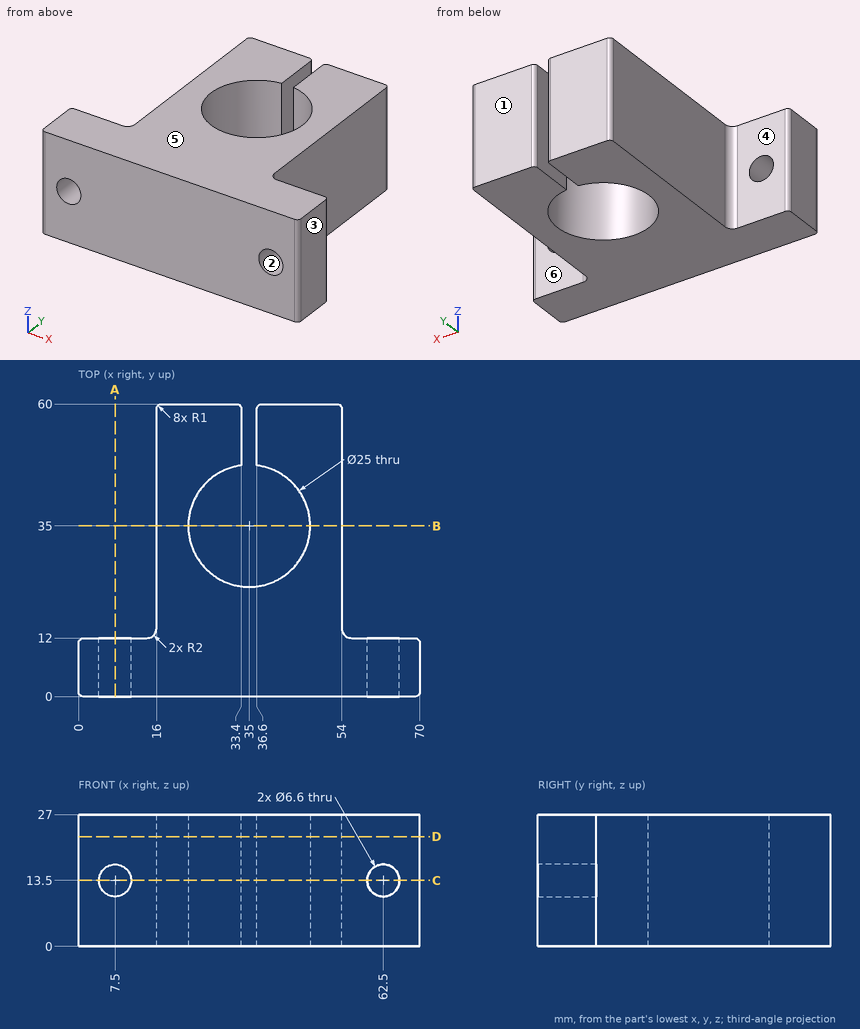
Study the drawing (mm; zero at the part's minimum x, y, z) and answer. A direction names the side the tool comes from. Give positions to 0.01 mm unless a question says otherwise; leave off trailing zeros. Loops run counter-clockwise (first coordinate to the right, second up) from the corner with the lowest first, then second, coordinate; pieces in that order, holes last. Notation, with made-up numbers: (55.25, 68.25) -> (75.25, 68.25) arc R19 ccw to (75.25, 79.25) -> close; hole circle Ø11 at (-36.5, 70). An arc over 180 degrees is marked (long way). Use a Markdown table: item, result. Add a question column.
1) The part is cut by section D-D, the plane z = 22.5. Determine the outline of the cut face in (x, y), plus the area to 3 significant figures.
2) The part is cut by section A-A, the plane x = 7.5. Determine the outline of the cut face in (y, z), plus the area to 3 significant figures.
3) The part is cut by section C-C, the plane z = 13.5. Count the separate pieces of the cut face and the enclosed holes in it, plus the area to 3 significant figures.
4) Each of these flat-tipped pins is pushed along its axis until it touches: P1, Ø5, axis at y = 17, z = 6, coming from the -X side; P2, Ø22.5, axis at x = 35, y = 35, coming from the +Z side; P3, Ø4, axis at x = 8, z = 18.5, coming from the +Y side; P4, Ø9.5, axis at y = 51.5, z = 13.5, coming from the +X side. Where does it stop, or does it pass through?
5) Which of the six approach directions +Z, -Z, +X, -X, +Y, -Y give full straight-line access (tool end or side, diameter ignored) to the marked faces 4, 5 and 6?
6) Consider line 1 along X through (y, z) = (4.25, 13.5); line 2 along X through (y, z) = (51, 6); line 3 along X through (y, z) = (7.5, 11.5). Determine where each line is inside the solid, lowest interval first.
7) The part is cut by section B-B, the plane y = 35. Determine the outline of the cut face in (x, z).
8) For a pull along X with two mould halves and no side action, classify the marked faces 1, 2 and 3 as +X half, -X half, draft (parallel to the pull), parting line (faces both ways), or undercut.
Reported:
| question | item | result |
|---|---|---|
| 1 | outline | (0, 1) arc R1 ccw to (1, 0) -> (69, 0) arc R1 ccw to (70, 1) -> (70, 11) arc R1 ccw to (69, 12) -> (56, 12) arc R2 cw to (54, 14) -> (54, 59) arc R1 ccw to (53, 60) -> (37.6, 60) arc R1 ccw to (36.6, 59) -> (36.6, 47.4) arc R12.5 cw (long way) to (33.4, 47.4) -> (33.4, 59) arc R1 ccw to (32.4, 60) -> (17, 60) arc R1 ccw to (16, 59) -> (16, 14) arc R2 cw to (14, 12) -> (1, 12) arc R1 ccw to (0, 11) -> close |
| 1 | area | 2,130 mm^2 |
| 2 | outline | (0, 0) -> (12, 0) -> (12, 10.2) -> (0, 10.2) -> close; (0, 16.8) -> (12, 16.8) -> (12, 27) -> (0, 27) -> close |
| 2 | area | 245 mm^2 |
| 3 | separate pieces | 3 |
| 3 | enclosed holes | 0 |
| 3 | area | 1,970 mm^2 |
| 4 | P1 | stops at x = 16 |
| 4 | P2 | passes through |
| 4 | P3 | stops at y = 12 |
| 4 | P4 | stops at x = 54 |
| 5 | face 4 | +Z, -Z, -X, +Y |
| 5 | face 5 | +Z, +X, -X, +Y, -Y |
| 5 | face 6 | +Z, -Z, +X, +Y |
| 6 | line 1 | x = 0 to 4.2, 10.8 to 59.2, 65.8 to 70 |
| 6 | line 2 | x = 16 to 33.4, 36.6 to 54 |
| 6 | line 3 | x = 0 to 4.88, 10.12 to 59.88, 65.12 to 70 |
| 7 | outline | (16, 0) -> (22.5, 0) -> (22.5, 27) -> (16, 27) -> close; (47.5, 0) -> (54, 0) -> (54, 27) -> (47.5, 27) -> close |
| 8 | face 1 | draft |
| 8 | face 2 | undercut |
| 8 | face 3 | +X half |
